from build123d import *

# Parameters (mm, degrees)
SKETCH1_W           = 219.61751697
SKETCH1_H           = 216.210653226
BOSS_EXTRUDE1_DEPTH = 10
CUT_EXTRUDE1_DEPTH  = 1
FILLET3_R           = 10
FILLET4_R           = 1


with BuildPart() as part:
    # Sketch1 → Boss-Extrude1 (new body)
    with BuildSketch(Plane(origin=(0, 0, 0), x_dir=(1, 0, 0), z_dir=(0, 1, 0))):
        with Locations((-13.550693969, -30.37560711)):
            Rectangle(SKETCH1_W, SKETCH1_H)
    extrude(amount=BOSS_EXTRUDE1_DEPTH)

    # Sketch2 → Cut-Extrude1 (cut)
    with BuildSketch(Plane(origin=(0, 10, 0), x_dir=(1, 0, 0), z_dir=(0, 1, 0))):
        with BuildLine():
            Line((34.100948693, -47.24181379), (34.100948693, -40.819164059))
            Line((34.100948693, -40.819164059), (6.100948693, -40.819164059))
            Line((6.100948693, -40.819164059), (6.100948693, -47.24181379))
            ThreePointArc((6.100948693, -47.24181379), (6.234923289, -47.74181379), (6.600948693, -48.107839194))
            Line((6.600948693, -48.107839194), (13.100948693, -51.860615944))
            Line((13.100948693, -51.860615944), (20.100948693, -55.902067828))
            Line((20.100948693, -55.902067828), (33.600948693, -48.107839194))
            ThreePointArc((33.600948693, -48.107839194), (33.966974097, -47.74181379), (34.100948693, -47.24181379))
        make_face()
        with BuildLine():
            Line((13.100948693, -59.943519712), (20.100948693, -55.902067828))
            Line((20.100948693, -55.902067828), (13.100948693, -51.860615944))
            Line((13.100948693, -51.860615944), (6.600948693, -55.613392693))
            ThreePointArc((6.600948693, -55.613392693), (6.234923289, -55.979418097), (6.100948693, -56.479418097))
            Line((6.100948693, -56.479418097), (6.100948693, -63.407621327))
            ThreePointArc((6.100948693, -63.407621327), (6.234923289, -63.907621327), (6.600948693, -64.273646731))
            Line((6.600948693, -64.273646731), (13.100948693, -68.026423481))
            Line((13.100948693, -68.026423481), (20.100948693, -63.984971597))
            Line((20.100948693, -63.984971597), (13.100948693, -59.943519712))
        make_face()
        with BuildLine():
            Line((20.100948693, -69.650779134), (20.100948693, -63.984971597))
            Line((20.100948693, -63.984971597), (13.100948693, -68.026423481))
            Line((13.100948693, -68.026423481), (6.600948693, -71.779200231))
            ThreePointArc((6.600948693, -71.779200231), (6.234923289, -72.145225634), (6.100948693, -72.645225634))
            Line((6.100948693, -72.645225634), (6.100948693, -80.150779134))
            Line((6.100948693, -80.150779134), (13.100948693, -76.10932725))
            Line((13.100948693, -76.10932725), (13.100948693, -69.650779134))
            ThreePointArc((13.100948693, -69.650779134), (13.504510857, -72.533823188), (14.684175934, -75.195250576))
            ThreePointArc((14.684175934, -75.195250576), (26.483992747, -79.74721697), (34.100948693, -69.650779134))
            Line((34.100948693, -69.650779134), (34.100948693, -55.902067828))
            Line((34.100948693, -55.902067828), (27.600948693, -59.654844578))
            ThreePointArc((27.600948693, -59.654844578), (27.234923289, -60.020869982), (27.100948693, -60.520869982))
            Line((27.100948693, -60.520869982), (27.100948693, -69.650779134))
            ThreePointArc((27.100948693, -69.650779134), (23.600948693, -73.150779134), (20.100948693, -69.650779134))
        make_face()
        with BuildLine():
            Line((13.100948693, -69.650779134), (13.100948693, -76.10932725))
            Line((13.100948693, -76.10932725), (14.684175934, -75.195250576))
            ThreePointArc((14.684175934, -75.195250576), (13.504510857, -72.533823188), (13.100948693, -69.650779134))
        make_face()
    extrude(amount=-CUT_EXTRUDE1_DEPTH, mode=Mode.SUBTRACT)

    # Fillet3
    fillet3_edges = [part.edges().sort_by_distance(p)[0] for p in [
        (-123.359452454, 5, -77.729719503),
        (96.258064516, 5, -77.729719503),
        (96.258064516, 5, 138.480933723),
        (-123.359452454, 5, 138.480933723),
    ]]
    fillet(fillet3_edges, radius=FILLET3_R)

    # Fillet4
    fillet4_edges = [part.edges().sort_by_distance(p)[0] for p in [
        (13.100948693, 9.5, 68.026423481),
        (13.100948693, 9.5, 51.860615944),
        (6.100948693, 9.5, 40.819164059),
        (34.100948693, 9.5, 40.819164059),
        (13.100948693, 9.5, 59.943519712),
        (20.100948693, 9.5, 63.984971597),
        (-13.550693969, 0, -77.729719503),
        (-13.550693969, 10, -77.729719503),
        (-123.359452454, 0, 30.37560711),
        (96.258064516, 0, 30.37560711),
        (-13.550693969, 0, 138.480933723),
        (93.329132328, 0, 135.552001535),
        (-120.430520266, 0, 135.552001535),
        (-120.430520266, 0, -74.800787315),
        (93.329132328, 0, -74.800787315),
        (96.258064516, 10, 30.37560711),
        (-123.359452454, 10, 30.37560711),
        (-13.550693969, 10, 138.480933723),
        (93.329132328, 10, 135.552001535),
        (-120.430520266, 10, 135.552001535),
        (-120.430520266, 10, -74.800787315),
        (93.329132328, 10, -74.800787315),
    ]]
    fillet(fillet4_edges, radius=FILLET4_R)


solid = part.part
Part model, mm, in its own coordinate system. A direction names the side the tool comes from. Coordinates: 2 decimals unless noted, no trailing zeros. Use a Markdown table: item, result. Add a question column.
Q1. Mould opens along X. For faces 3 (the flat face through (-15, 0, 29)), 4 (the flat face through (19.9, 9, 55.8)), 5 (the cylindrical face through (-120.51, 5.06, -74.72)) say: +X half, -X half, draft (parallel to the pull), parting line (faces both ways), or undercut.
Q2. Probe L1, parallel to X at y = 9, z = -68; L2, parallel to Z at x = 78.5, y = 0.75; L3, parallel to X at y = 9.25, z = 52.5. List the from-to ranges inside material, lowest first.
Q3. Which spindle directions (+Z, -Z, +X, -X, +Y, -Y) get a long thin tool onto all of the face, cutting with end or side? Do faces 1 (the flat face through (-123.359, 5, 32)), 2 (the cylindrical face through (26.3, 9.5, 79.8)). Say none if no direction does.
Q4. Pin check, flat tips, straight feed: P1, Ø0.8, axis at y = 9.5, z = 66.5, coming from the +X side; P2, Ø0.8, axis at y = 9.5, z = 62, coming from the -X side; P3, Ø0.5, axis at y = 9.5, z = 76, coming from the +X side. Stop position of each tip, or through.
Worked out:
| question | item | result |
|---|---|---|
| 1 | face 3 | draft |
| 1 | face 4 | undercut |
| 1 | face 5 | -X half |
| 2 | L1 | x = -123.36 to 96.25 |
| 2 | L2 | z = -77.7 to 138.45 |
| 2 | L3 | x = -123.33 to 11.87, 25.99 to 96.23 |
| 3 | face 1 | +Z, -Z, -X, +Y, -Y |
| 3 | face 2 | +Y |
| 4 | P1 | stops at x = 96.25 |
| 4 | P2 | stops at x = -123.35 |
| 4 | P3 | stops at x = 96.23 |
